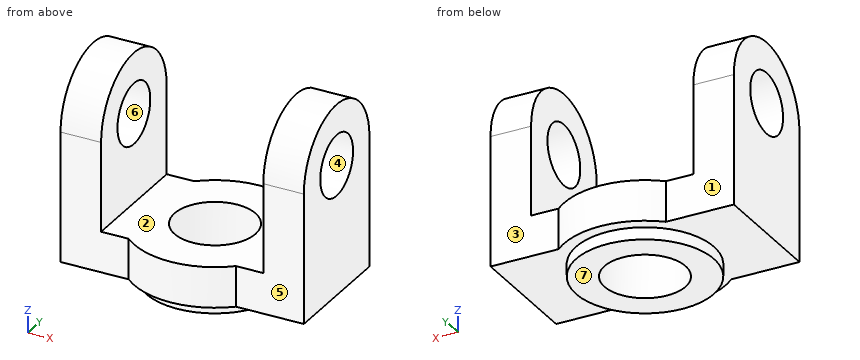
```python
from build123d import *

# Parameters (mm, degrees)
F0_R     = 10
F1_DEPTH = 10
F2_R     = 17
F2_R_2   = 10
F3_DEPTH = 3
F4_R     = 7.5
F5_DEPTH = 10
F6_R     = 7.5
F7_DEPTH = 10


with BuildPart() as f1:
    # F0 (on Top) → F1 (new body)
    with BuildSketch(Plane.XY):
        with BuildLine():
            ThreePointArc((-13.2287565553, -15), (-20, 0), (-13.2287565553, 15))
            Line((-13.2287565553, 15), (-30, 15))
            Line((-30, 15), (-30, -15))
            Line((-30, -15), (-13.2287565553, -15))
        make_face()
        with BuildLine():
            Line((-13.2287565553, 15), (13.2287565553, 15))
            ThreePointArc((13.2287565553, 15), (0, 20), (-13.2287565553, 15))
        make_face()
        with BuildLine():
            ThreePointArc((20, 0), (18.2287565553, 8.2287565553), (13.2287565553, 15))
            Line((13.2287565553, 15), (-13.2287565553, 15))
            ThreePointArc((-13.2287565553, 15), (-20, 0), (-13.2287565553, -15))
            Line((-13.2287565553, -15), (13.2287565553, -15))
            ThreePointArc((13.2287565553, -15), (18.2287565553, -8.2287565553), (20, 0))
        make_face()
        Circle(F0_R, mode=Mode.SUBTRACT)
        with BuildLine():
            Line((30, -15), (30, 15))
            Line((30, 15), (13.2287565553, 15))
            ThreePointArc((13.2287565553, 15), (18.2287565553, 8.2287565553), (20, 0))
            ThreePointArc((20, 0), (18.2287565553, -8.2287565553), (13.2287565553, -15))
            Line((13.2287565553, -15), (30, -15))
        make_face()
        with BuildLine():
            ThreePointArc((-13.2287565553, -15), (0, -20), (13.2287565553, -15))
            Line((13.2287565553, -15), (-13.2287565553, -15))
        make_face()
    extrude(amount=F1_DEPTH)

    # F2 (on face) → F3 (join)
    with BuildSketch(Plane(origin=(0, 0, 0), x_dir=(1, 0, 0), z_dir=(0, 0, -1))):
        Circle(F2_R)
        Circle(F2_R_2, mode=Mode.SUBTRACT)
    extrude(amount=F3_DEPTH)

    # F4 (on face) → F5 (join)
    with BuildSketch(Plane.YZ.offset(30)):
        with BuildLine():
            Line((-15, 32), (-15, 10))
            Line((-15, 10), (15, 10))
            Line((15, 10), (15, 32))
            ThreePointArc((15, 32), (0, 47), (-15, 32))
        make_face()
        with Locations((0, 32)):
            Circle(F4_R, mode=Mode.SUBTRACT)
    extrude(amount=-F5_DEPTH)

    # F6 (on face) → F7 (join)
    with BuildSketch(Plane(origin=(-30, 0, 0), x_dir=(0, -1, 0), z_dir=(-1, 0, 0))):
        with BuildLine():
            Line((-15, 10), (15, 10))
            Line((15, 10), (15, 32))
            ThreePointArc((15, 32), (0, 47), (-15, 32))
            Line((-15, 32), (-15, 10))
        make_face()
        with Locations((0, 32)):
            Circle(F6_R, mode=Mode.SUBTRACT)
    extrude(amount=-F7_DEPTH)


solid = f1.part
```
Geometry check sheet. Reference: the model listing, model coordinates, mm. Face numbers are marked on the shaded views. A direction names the side the tool comes from. Round coordinates to 2 decimals unless told otherwise and drop trailing zeros. Loops run counter-clockwise (first coordinate to the right, second up) from the corner with the lowest first, then second, coordinate; pieces in that order, holes last. Notation, with made-up numbers: M 6.25,-29 L 37.25,-29 A14 cw 37.25,-5 Z; hole C 83,49.5 d11. An arc over 180 degrees is marked long. Return JSON: item names as keys, results as strings. Group by question number.
(1) Section check B-B, the plane y = 0. Enter the section's corners in (x, z).
(2) Section check D-D, the plane z = 34.5. Enter the section's corners in (x, y), and give its area (3 significant figures).
(3) Mould release check, pull along Z, two halves, no side actions. Record for the marked faces 4, 5, 6 and 7: pulls with the +Z half, pulls with the -Z half, needs draft (parallel to the pull), parting line crosses it, or undercut.
(4) Section check A-A, the plane z = 18.5. Enter the section's corners in (x, y).
(5) Scan lines: line 1 along X through (y, z) = (-9, 18); line 2 along X through (y, z) = (0, 2); line 3 along Z through (x, y) = (25.75, 0). Record each from-to range of solid material in increasing order. Write a range as [from, to].
(6) Set-up check for the marked faces 1, 2 and 3: record each of +Z, -Z, +X, -X, +Y, -Y from which the full face is reachable in a straight line by a thin tool's end or side.
(7) Go/stop test with flat-tipped pins: pin 1 (5 mm diameter, centred on x = -21, z = 17, fed in from +Y); pin 2 (4 mm diameter, centred on x = -8, z = 6.5, fed in from -Y); pin 3 (10 mm diameter, centred on x = 12.5, z = 31, fed in from -Y); pin 4 (18.5 mm diameter, centred on x = 18, z = 12.5, fed in from +Y). Record where each tip stops, or that it passes through.
(8) Section check C-C, the plane x = 0. Enter the section's corners in (y, z), and give its area (3 significant figures).
Data:
{
 "1": {"outline": "M -30,0 L -17,0 L -17,-3 L -10,-3 L -10,10 L -20,10 L -20,24.5 L -30,24.5 Z; M -30,39.5 L -20,39.5 L -20,47 L -30,47 Z; M 10,-3 L 17,-3 L 17,0 L 30,0 L 30,24.5 L 20,24.5 L 20,10 L 10,10 Z; M 20,39.5 L 30,39.5 L 30,47 L 20,47 Z"},
 "2": {"outline": "M -30,-14.79 L -20,-14.79 L -20,-7.07 L -30,-7.07 Z; M -30,7.07 L -20,7.07 L -20,14.79 L -30,14.79 Z; M 20,-14.79 L 30,-14.79 L 30,-7.07 L 20,-7.07 Z; M 20,7.07 L 30,7.07 L 30,14.79 L 20,14.79 Z", "area": "309 mm²"},
 "3": {"face 4": "undercut", "face 5": "needs draft", "face 6": "undercut", "face 7": "pulls with the -Z half"},
 "4": {"outline": "M -30,-15 L -20,-15 L -20,15 L -30,15 Z; M 20,-15 L 30,-15 L 30,15 L 20,15 Z"},
 "5": {"line 1": "[-30, -20], [20, 30]", "line 2": "[-30, -10], [10, 30]", "line 3": "[0, 24.5], [39.5, 47]"},
 "6": {"face 1": "+Z, -Z, -X, +Y", "face 2": "+Z, +Y, -Y", "face 3": "+Z, -Z, +X, +Y"},
 "7": {"pin 1": "y = 15", "pin 2": "y = -19.08", "pin 3": "through", "pin 4": "y = 17.81"},
 "8": {"outline": "M -20,0 L -17,0 L -17,-3 L -10,-3 L -10,10 L -20,10 Z; M 10,-3 L 17,-3 L 17,0 L 20,0 L 20,10 L 10,10 Z", "area": "242 mm²"}
}
